Drawing for the job (mm, zero at the part's lowest x, y, z). A direction names the side the tool comes from. Give positions to 0.01 mm unless a question says otherwise; leave off trailing zeros. Order: outer loops, then holes, each group sorted by start corner. A loop starts at its lowest first (then second) coordinate and runs counter-clockwise, first axis right, second up. Notation, with made-up numbers: (9, -34) - (49, -34) arc R16 cw to (49, -19) - close; hole circle Ø7 at (-14, -17). An arc over 180 degrees is marked (long way). Use CSV: the item, a comma, the result in double quotes. Start each with the question number.
(1) Drop a flat-ended pin along its axis: pin 1 Ø1 at (x, y) = (6.5, 1.5) entering from -Z. Give the stop position or say it passes through.
(2) Tool access for the marked faces 5, 6 and 7: list every direction of +Z, -Z, +X, -X, +Y, -Y with a clear straight run to the whole face (end or side of a thin tool).
(3) Band-saw the part on A-A, the plane z = 14.5. Give the cut face in (x, y).
(4) Pull direction X, two halves, no side cores. Call the marked faces 1, 2, 3 and 4: +X half, -X half, draft (parallel to the pull), parting line (faces both ways), or undercut.
(5) Band-saw the part on B-B, the plane y = 1.15. Give the cut face in (x, z).
(6) Band-saw the part on D-D, the plane x = 11.25. Give the cut face in (y, z), then the cut area to 3 significant figures.
(7) Band-saw the part on C-C, the plane x = 15.75. Give the cut face in (y, z), then the cut area to 3 significant figures.
(8) Probe L1, parallel to X at y = 1.25, z = 2.5; L2, parallel to X at y = 2.6, z = 13.5; L3, parallel to Z at x = 1.25, y = 0.5. List the from-to ranges inside material, lowest first.
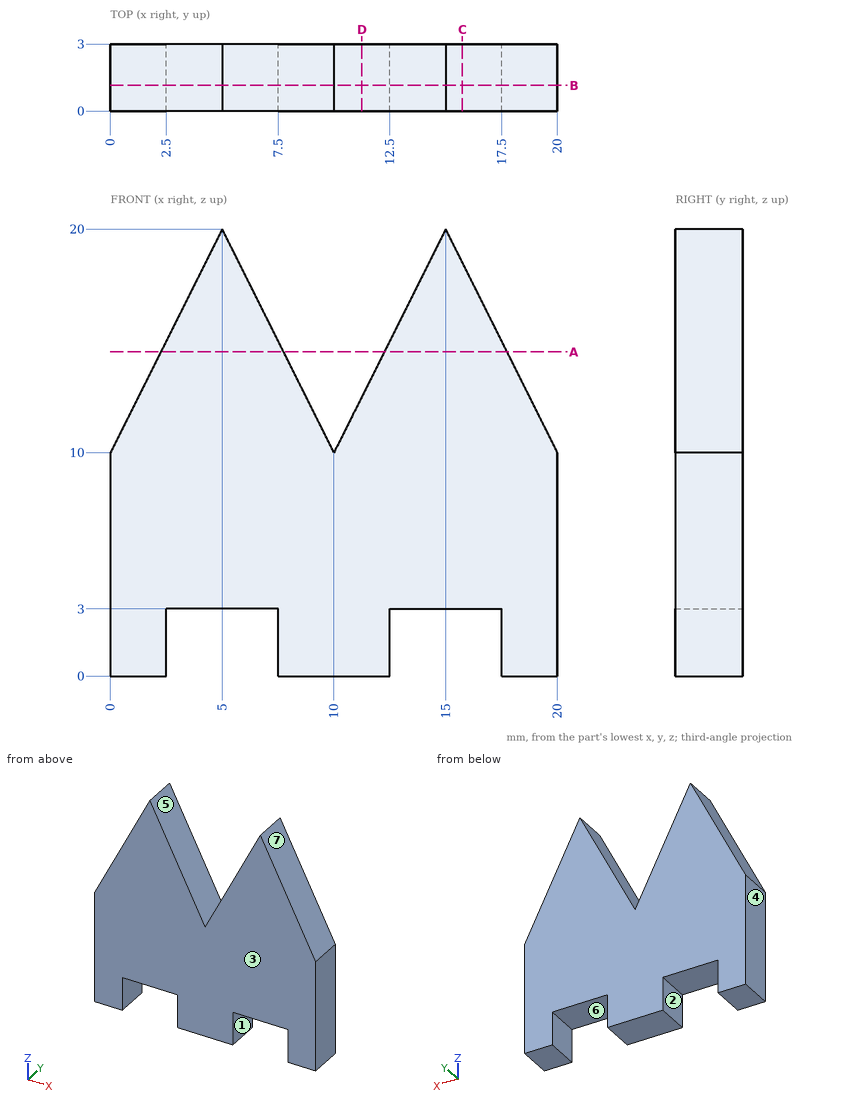
Answer block:
1,pin 1,"stops at z = 3"
2,face 5,"+Z, +Y, -Y"
2,face 6,"-Z, +Y, -Y"
2,face 7,"+Z, +X, +Y, -Y"
3,outline,"(2.25, 0) - (7.75, 0) - (7.75, 3) - (2.25, 3) - close; (12.25, 0) - (17.75, 0) - (17.75, 3) - (12.25, 3) - close"
4,face 1,"undercut"
4,face 2,"undercut"
4,face 3,"draft"
4,face 4,"-X half"
5,outline,"(0, 0) - (2.5, 0) - (2.5, 3) - (7.5, 3) - (7.5, 0) - (12.5, 0) - (12.5, 3) - (17.5, 3) - (17.5, 0) - (20, 0) - (20, 10) - (15, 20) - (10, 10) - (5, 20) - (0, 10) - close"
6,outline,"(0, 0) - (3, 0) - (3, 12.5) - (0, 12.5) - close"
6,area,"37.5 mm2"
7,outline,"(0, 3) - (3, 3) - (3, 18.5) - (0, 18.5) - close"
7,area,"46.5 mm2"
8,L1,"x = 0 to 2.5, 7.5 to 12.5, 17.5 to 20"
8,L2,"x = 1.75 to 8.25, 11.75 to 18.25"
8,L3,"z = 0 to 12.5"
